Geometry check sheet. Reference: the model listing, model coordinates, mm. Face numbers are marked on the shaded views. Coordinates: 2 decimals unless noted, no trailing zeros. Loops run counter-clockwise (first coordinate to the right, second up) from the corner with the lowest first, then second, coordinate; pieces in that order, holes last. Notation, with made-up numbers: (11.5, -11.5) - (26.5, -11.5) arc R10 cw to (26.5, 4.5) - close; hole circle Ø1 at (-19, 48.25). An arc over 180 degrees is marked (long way). Write each question's results on one line, items separated by ' | '. Start each with the question number.
(1) Sectioned sample at A-A (z = -7). Enter the section's corners in (x, y), plus the area to 3 significant figures.
(2) Go/stop test with flat-tipped pins: pin 1 Ø8 at (y, z) = (-4.5, -4) entering from +X; pin 2 Ø10 at (y, z) = (-7, -3) entering from +X; pin 3 Ø10 at (x, z) = (4, -6) entering from +Y. Record where each tip stops, or that it passes through.
(3) Sectioned sample at B-B (z = 3). Enter the section's corners in (x, y), plus the area to 3 significant figures.
(4) Material ranges on probe 1 along Y at (x, z) = (0, 1.8); probe 2 along Z at (x, y) = (-0.25, -3.5); probe 3 along X at (y, z) = (-1, 0.75), recorded low to high.
(5) Mould release check, pull along Y, two halves, no side actions. Record for the marked faces 1, 2, 3 and 4: pulls with the +Y half, pulls with the -Y half, needs draft (parallel to the pull), parting line crosses it, or undercut.
from build123d import *

# Parameters (mm, degrees)
F3_DEPTH = 7.62
F5_R     = 5
F6_R     = 0.99999
F7_R     = 0.5


# Not quite as in the source:
# - a fillet or chamfer that OpenCascade refuses, or shapes differently, is made with other operations: its cross-section is extruded or revolved along the edge and cut away or added
# - a fillet or chamfer is up to 0.001 mm smaller than in the source, because OpenCascade refuses the exact size


with BuildPart() as f1:
    # F0 (on Front) → F1 (revolve)
    with BuildSketch(Plane.XZ):
        Polygon((8, 5), (8, 0), (0, 0), (0, -12), (7, -12), (7, -5), (10, -5), (10, 5), align=None)
    revolve(axis=Axis((0, 0, -6), (0, 0, 1)))

    # F2 (on face) → F3 (cut)
    with BuildSketch(Plane(origin=(0, 0, -12), x_dir=(1, 0, 0), z_dir=(0, 0, -1))):
        Polygon((1.1547005384, 2), (-1.1547005384, 2), (-2.3094010768, 0), (-1.1547005384, -2), (1.1547005384, -2), (2.3094010768, 0), align=None)
    extrude(amount=-F3_DEPTH, mode=Mode.SUBTRACT)

    # F4: fillet of radius 5 on 1 edges, made by hand

    # F4_s1 → F4_t2 (revolve)
    with BuildSketch(Plane.XZ):
        with BuildLine():
            ThreePointArc((10, -5), (7.8166998673, -6.8439629074), (7, -9.582575695))
            Line((7, -9.582575695), (7, -5))
            Line((7, -5), (10, -5))
        make_face()
    revolve(axis=Axis((0, 0, -5), (0, 0, 1)))

    # F5
    f5_edges = [f1.edges().sort_by_distance(p)[0] for p in [
        (-10, 0, -5),
    ]]
    fillet(f5_edges, radius=F5_R)

    # F6 (radius 1 in the source; OpenCascade refuses exactly that, so slightly less here)
    f6_edges = [f1.edges().sort_by_distance(p)[0] for p in [
        (-10, 0, 5),
        (-8, 0, 5),
        (-7, 0, -12),
    ]]
    fillet(f6_edges, radius=F6_R)

    # F7
    f7_edges = [f1.edges().sort_by_distance(p)[0] for p in [
        (-2.309401, 0, -8.19),
        (-1.154701, -2, -8.19),
        (1.154701, -2, -8.19),
        (2.309401, 0, -8.19),
        (1.154701, 2, -8.19),
        (-1.154701, 2, -8.19),
    ]]
    fillet(f7_edges, radius=F7_R)


solid = f1.part
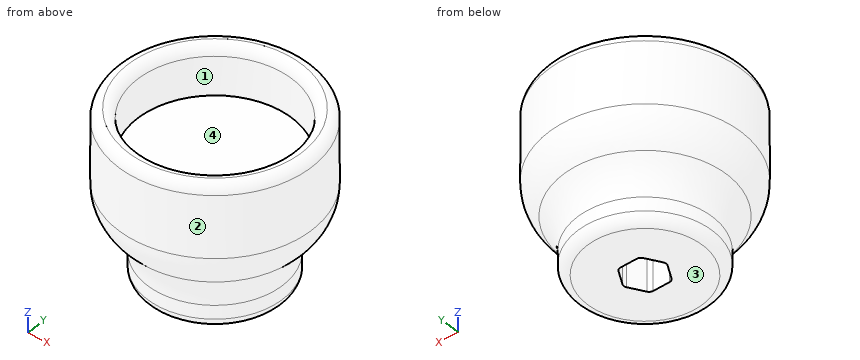
Outcome:
1) outline: circle Ø15.44 at (0, 0); hole (-2.17, -0.25) - (-1.3, -1.75) arc R0.5 ccw to (-0.87, -2) - (0.87, -2) arc R0.5 ccw to (1.3, -1.75) - (2.17, -0.25) arc R0.5 ccw to (2.17, 0.25) - (1.3, 1.75) arc R0.5 ccw to (0.87, 2) - (-0.87, 2) arc R0.5 ccw to (-1.3, 1.75) - (-2.17, 0.25) arc R0.5 ccw to start | area: 173 mm2
2) pin 1: stops at x = 9.97 | pin 2: stops at x = 9.79 | pin 3: stops at y = 9.99
3) outline: circle Ø20 at (0, 0); hole circle Ø16 at (0, 0) | area: 113 mm2
4) probe 1: y = -10 to -8, 8 to 10 | probe 2: z = -12 to 0 | probe 3: x = -9.95 to -7.94, 7.94 to 9.95
5) face 1: undercut | face 2: parting line crosses it | face 3: needs draft | face 4: undercut
